Read the model definition and answer for the solid it produces. Units are mm, in the model's axes. A direction names the side the tool comes from. Coordinates: 2 decimals unless noted, no trailing zeros. Loops run counter-clockwise (first coordinate to the right, second up) from the corner with the lowest first, then second, coordinate; pieces in that order, holes last. Notation, with made-up numbers: (75.25, 59) -> (118.25, 59) arc R22 ccw to (118.25, 97) -> close; hole circle Ø5 at (41, -4.5). An arc over 180 degrees is marked (long way). Answer in a Markdown table with one row per item.
Autodesk Inventor part; units mm, degrees
ref_plane "YZ Plane" through (0, 0, 0) normal (1, 0, 0) x (0, 1, 0)
ref_plane "XZ Plane" through (0, 0, 0) normal (0, 1, 0) x (-1, 0, 0)
ref_plane "XY Plane" through (0, 0, 0) normal (0, 0, 1) x (1, 0, 0)
sketch "スケッチ1" plane through (0, 0, 0) normal (0, 0, 1) x (1, 0, 0)
  line L0 (0, 0) -> (50, 0)
  line L1 (50, 0) -> (50, 10)
  line L2 (50, 10) -> (0, 10)
  line L3 (0, 10) -> (0, 0)
  dimension "d0" = 50
  dimension "d1" = 10
extrude "押し出し1" add sketch "スケッチ1" along normal blind 2.5
sketch "スケッチ2" plane through (0, 0, 2.5) normal (0, 0, 1) x (1, 0, 0)
  line L0 (10, -2.5) -> (0, -2.5)
  line L1 (10, 0) -> (10, -2.5)
  line L2 (0, 0) -> (10, 0)
  line L3 (0, 0) -> (0, -2.5)
  line L4 (42.7436, -2.5) -> (32.7436, -2.5)
  line L5 (42.7436, 0) -> (42.7436, -2.5)
  line L6 (32.7436, 0) -> (42.7436, 0)
  line L7 (32.7436, 0) -> (32.7436, -2.5)
  line L8 (42.7436, 0) -> (42.7436, 10)
  line L9 (50, 0) -> (50, 10)
  line L10 (50, 10) -> (0, 10)
  line L11 (0, 10) -> (0, 0)
  line L12 (0, 0) -> (50, 0)
extrude "押し出し2" cut sketch "スケッチ2" against normal through all contours L8 L10 L9 L12
sketch "スケッチ3" plane through (0, 0, 2.5) normal (0, 0, 1) x (1, 0, 0)
  line L0 (10, -2.5) -> (0, -2.5)
  line L1 (10, 0) -> (10, -2.5)
  line L2 (0, 0) -> (10, 0)
  line L3 (0, 0) -> (0, -2.5)
  line L4 (42.7436, -2.5) -> (32.7436, -2.5)
  line L5 (42.7436, 0) -> (42.7436, -2.5)
  line L6 (32.7436, 0) -> (42.7436, 0)
  line L7 (32.7436, 0) -> (32.7436, -2.5)
extrude "押し出し3" add sketch "スケッチ3" against normal up to surface (2.5 mm away)
properties part number "皿_壁"
1. A cutting plane is placed at C-C on x = 26. Give the vertices of the cut face in (y, z).
A:
| item | result |
|---|---|
| outline | (0, 0) -> (10, 0) -> (10, 2.5) -> (0, 2.5) -> close |
2. The mould has two halves that part along X. Classify faces 1 (the flat face through (22, 10, 1)), 2 (the flat face through (0, 4, 1)), 3 (the flat face through (32.744, -1, 1)): pulls with the +X half, pulls with the -X half, needs draft (parallel to the pull), parting line crosses it, or undercut.
A:
| item | result |
|---|---|
| face 1 | needs draft |
| face 2 | pulls with the -X half |
| face 3 | undercut |
3. Given pin 1 Ø0.8 at (x, z) = (21, 1) entering from -Y; pin 2 Ø2 at (x, y) = (30.5, 6) entering from -Z, each flat-ended and moving along its own axis, determine where each tip first touches the part or whether it passes through.
A:
| item | result |
|---|---|
| pin 1 | stops at y = 0 |
| pin 2 | stops at z = 0 |
4. A cutting plane is placed at B-B on z = 1.95. Give the vertices of the cut face in (x, y).
A:
| item | result |
|---|---|
| outline | (0, -2.5) -> (10, -2.5) -> (10, 0) -> (32.74, 0) -> (32.74, -2.5) -> (42.74, -2.5) -> (42.74, 10) -> (0, 10) -> close |
5. Find the intervals of material crossed by probe 1 along X at (y, z) = (-0.25, 1.2); probe 2 along Y at (x, z) = (24.5, 0.8), in increasing order.
A:
| item | result |
|---|---|
| probe 1 | x = 0 to 10, 32.74 to 42.74 |
| probe 2 | y = 0 to 10 |
6. A tool of negligible diameter and unlimited length cuts with its end or side. For faces 4 (the flat face through (21, 0, 1)), 5 (the flat face through (42.744, 4, 1)), from which of +Z, -Z, +X, -X, +Y, -Y can it reach the whole face along a straight path? Write none if from no direction.
A:
| item | result |
|---|---|
| face 4 | +Z, -Z, -Y |
| face 5 | +Z, -Z, +X, +Y, -Y |
7. A cutting plane is placed at A-A on y = -0.75. Give the vertices of the cut face in (x, z).
A:
| item | result |
|---|---|
| outline | (0, 0) -> (10, 0) -> (10, 2.5) -> (0, 2.5) -> close; (32.74, 0) -> (42.74, 0) -> (42.74, 2.5) -> (32.74, 2.5) -> close |
